Can you work these out from the model? Positions are in its coordinate system, mm. Coordinates: 2 decimals unless noted, no trailing zeros. Loops run counter-clockwise (first coordinate to the right, second up) from the corner with the lowest first, then second, coordinate; pieces in that order, holes last. Notation, with made-up numbers: (88.25, 62.25) -> (111.25, 62.25) arc R21 ccw to (111.25, 73.25) -> close; hole circle Ø8 at (64.5, -5). An arc over 180 degrees is marked (long way). Use one line per item in the form item = value. Start each with the question number.
(1) I need wall thicknesses on line 1 (Y direction, x = -25.4, z = 0.9); line 2 (Y direction, x = -5.5, z = 0.1). Which ranges of each line are inside material? Lowest first, please. Write a range as [from, to].
(2) Thinking about a two-plate mould opening in X: for faces 1 (the flat face through (35.585, 0, 1)), 2 (the cylindrical face through (4.74, 14.64, 0.8)), 3 (the flat face through (0, 0, 0)), which applies, released by +X, released by -X, zero draft, split by the parting line, or undercut?
(3) Imagine slicing it at A-A (x = 15.24). List the corners of the cut face in (y, z) for me.
(4) I'm going to push flat-ended pins straight in: pin 1 (3.5 mm diameter, centred on x = 25.4, y = 15.72, fed in from +Z); pin 2 (1.4 mm diameter, centred on x = -25.4, y = 15.72, fed in from -Z). Where does each tip first touch, or does it pass through?
(5) Imagine slicing it at B-B (z = 0.4). State how many separate pieces and enclosed holes the cut face has, plus the area to 3 significant figures.
```python
from build123d import *

# Parameters (mm, degrees)
SKETCH1_W           = 71.1708
SKETCH1_H           = 35.2425
BOSS_EXTRUDE1_DEPTH = 1.5875
LPATTERN1_COUNT     = 6
LPATTERN1_PITCH     = 10.16


with BuildPart() as part:
    # Sketch1 → Boss-Extrude1 (new body)
    with BuildSketch(Plane.XY):
        Rectangle(SKETCH1_W, SKETCH1_H)
    extrude(amount=BOSS_EXTRUDE1_DEPTH)

    # Sketch3 → #2 Clearance Hole1 (revolve, cut)
    with BuildSketch(Plane(origin=(-25.4, 15.71625, 1.5875), x_dir=(0, -1, 0), z_dir=(1, 0, 0))):
        Polygon((0, 0), (0, 3.854152758), (1.1303, 3.175), (1.1303, 0), align=None)
    f_2_clearance_hole1 = revolve(axis=Axis((-25.4, 15.71625, 7.9375), (0, 0, -1)), mode=Mode.SUBTRACT)

    # LPattern1: #2 Clearance Hole1 ×6
    with Locations(*[(i * LPATTERN1_PITCH, 0, 0) for i in range(1, LPATTERN1_COUNT)]):
        add(f_2_clearance_hole1, mode=Mode.SUBTRACT)

    # Mirror1: #2 Clearance Hole1 across plane
    add(f_2_clearance_hole1.mirror(Plane.ZX), mode=Mode.SUBTRACT)

    # Mirror1 copy 1 sketch → Mirror1 copy 1 (revolve, cut)
    with BuildSketch(Plane(origin=(-15.24, -15.71625, 1.5875), x_dir=(0, 1, 0), z_dir=(1, 0, 0))):
        Polygon((0, 0), (0, -3.854152758), (1.1303, -3.175), (1.1303, 0), align=None)
    revolve(axis=Axis((-15.24, -15.71625, 7.9375), (0, 0, 1)), mode=Mode.SUBTRACT)

    # Mirror1 copy 2 sketch → Mirror1 copy 2 (revolve, cut)
    with BuildSketch(Plane(origin=(-5.08, -15.71625, 1.5875), x_dir=(0, 1, 0), z_dir=(1, 0, 0))):
        Polygon((0, 0), (0, -3.854152758), (1.1303, -3.175), (1.1303, 0), align=None)
    revolve(axis=Axis((-5.08, -15.71625, 7.9375), (0, 0, 1)), mode=Mode.SUBTRACT)

    # Mirror1 copy 3 sketch → Mirror1 copy 3 (revolve, cut)
    with BuildSketch(Plane(origin=(5.08, -15.71625, 1.5875), x_dir=(0, 1, 0), z_dir=(1, 0, 0))):
        Polygon((0, 0), (0, -3.854152758), (1.1303, -3.175), (1.1303, 0), align=None)
    revolve(axis=Axis((5.08, -15.71625, 7.9375), (0, 0, 1)), mode=Mode.SUBTRACT)

    # Mirror1 copy 4 sketch → Mirror1 copy 4 (revolve, cut)
    with BuildSketch(Plane(origin=(15.24, -15.71625, 1.5875), x_dir=(0, 1, 0), z_dir=(1, 0, 0))):
        Polygon((0, 0), (0, -3.854152758), (1.1303, -3.175), (1.1303, 0), align=None)
    revolve(axis=Axis((15.24, -15.71625, 7.9375), (0, 0, 1)), mode=Mode.SUBTRACT)

    # Mirror1 copy 5 sketch → Mirror1 copy 5 (revolve, cut)
    with BuildSketch(Plane(origin=(25.4, -15.71625, 1.5875), x_dir=(0, 1, 0), z_dir=(1, 0, 0))):
        Polygon((0, 0), (0, -3.854152758), (1.1303, -3.175), (1.1303, 0), align=None)
    revolve(axis=Axis((25.4, -15.71625, 7.9375), (0, 0, 1)), mode=Mode.SUBTRACT)


solid = part.part
```
Worked out:
q1.line_1 = [-17.62, -16.85], [-14.59, 14.59], [16.85, 17.62]
q1.line_2 = [-17.62, -16.77], [-14.67, 14.67], [16.77, 17.62]
q2.face_1 = released by +X
q2.face_2 = undercut
q2.face_3 = zero draft
q3.outline = (-17.62, 0) -> (-16.85, 0) -> (-16.85, 1.59) -> (-17.62, 1.59) -> close; (-14.59, 0) -> (14.59, 0) -> (14.59, 1.59) -> (-14.59, 1.59) -> close; (16.85, 0) -> (17.62, 0) -> (17.62, 1.59) -> (16.85, 1.59) -> close
q4.pin_1 = 1.59
q4.pin_2 = through
q5.separate_pieces = 1
q5.enclosed_holes = 12
q5.area = 2,460 mm2
